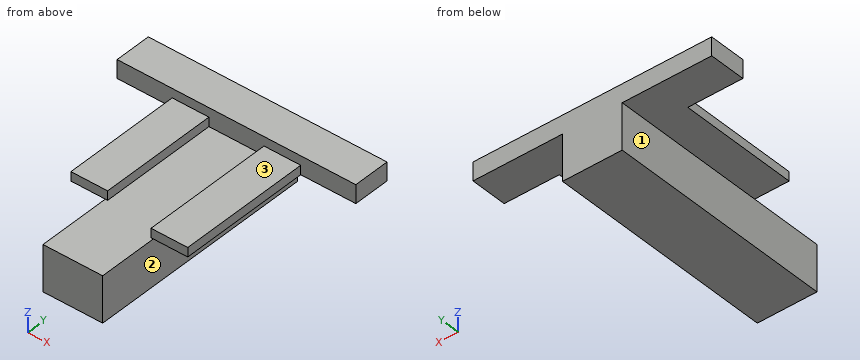
```python
from build123d import *

# Parameters (mm, degrees)
F0_W     = 82.55
F0_H     = 12.7
F1_DEPTH = 6.35
F2_W     = 12.7
F2_H     = 53.975
F2_H_2   = 58.7375
F3_DEPTH = 3.175
F4_W     = 20.6375
F4_H     = 79.375
F5_DEPTH = 15.875


with BuildPart() as f1:
    # F0 (on Top) → F1 (new body)
    with BuildSketch(Plane.XY):
        with Locations((0, 73.025)):
            Rectangle(F0_W, F0_H)
    extrude(amount=F1_DEPTH)

    # F2 (on face) → F3 (join)
    with BuildSketch(Plane(origin=(0, 0, 0), x_dir=(1, 0, 0), z_dir=(0, 0, -1))):
        with Locations((-15.875, -52.3875)):
            Rectangle(F2_W, F2_H)
        with Locations((15.875, -50.00625)):
            Rectangle(F2_W, F2_H_2)
    extrude(amount=-F3_DEPTH)

    # F4 (on face) → F5 (join)
    with BuildSketch(Plane(origin=(0, 0, 0), x_dir=(1, 0, 0), z_dir=(0, 0, -1))):
        with Locations((0, -39.6875)):
            Rectangle(F4_W, F4_H)
    extrude(amount=F5_DEPTH)


solid = f1.part
```
Geometry check sheet. Reference: the model listing, model coordinates, mm. Face numbers are marked on the shaded views. A direction names the side the tool comes from. Coordinates: 2 decimals unless noted, no trailing zeros. Order: outer loops, then holes, each group sorted by start corner. A loop starts at its lowest first (then second) coordinate and runs counter-clockwise, first axis right, second up.
Item 1: Section check B-B (y = 65.5). Enter the section's corners in (x, z) (3 decimals).
Item 2: Tool access check on the marked faces 1, 2 and 3. Record the directions out of +Z, -Z, +X, -X, +Y, -Y that give a thin tool (end or side, any length) a straight path to the whole face; none if there is none.
Item 3: Scan lines: line 1 along X through (y, z) = (61, -14); line 2 along Z through (x, y) = (10.5, 44) (3 decimals); line 3 along Y through (x, z) = (22, 4.75) (3 decimals). Record each from-to range of solid material in increasing order.
Item 4: Section check A-A (z = 2). Enter the section's corners in (x, y) (1 decimal).
Item 5: Section check C-C (x = -15). Enter the section's corners in (y, z) (3 decimals), plus the area to 3 significant figures.
Item 6: Depth check by flat-ended pin: pin 1 (5 mm diameter, centred on y = 29.5, z = -4.5, fed in from -X); pin 2 (14 mm diameter, centred on x = 16.5, y = 38, fed in from +Z) (3 decimals); pin 3 (1 mm diameter, centred on y = 50.5, z = 1.5, fed in from -X) (3 decimals). Enter the tip coordinate at first touch or a pass-through.
Check sheet entries:
1. outline: (-22.225, 0) - (-10.319, 0) - (-10.319, -15.875) - (10.319, -15.875) - (10.319, 0) - (22.225, 0) - (22.225, 3.175) - (9.525, 3.175) - (9.525, 0) - (-9.525, 0) - (-9.525, 3.175) - (-22.225, 3.175) - close
2. face 1: -Z, -X, +Y, -Y
2. face 2: -Z, +X, +Y, -Y
2. face 3: +Z, +X, -X, -Y
3. line 1: x = -10.32 to 10.32
3. line 2: z = 0 to 3.175
3. line 3: y = 66.675 to 79.375
4. outline: (-41.3, 66.7) - (-22.2, 66.7) - (-22.2, 25.4) - (-9.5, 25.4) - (-9.5, 66.7) - (9.5, 66.7) - (9.5, 20.6) - (22.2, 20.6) - (22.2, 66.7) - (41.3, 66.7) - (41.3, 79.4) - (-41.3, 79.4) - close
5. outline: (25.4, 0) - (79.375, 0) - (79.375, 6.35) - (66.675, 6.35) - (66.675, 3.175) - (25.4, 3.175) - close
5. area: 212 mm2
6. pin 1: stops at x = -10.32
6. pin 2: stops at z = 3.175
6. pin 3: stops at x = -22.225
